Input: part model. Units: mm. Frame: model coordinates. Face numbers are marked on the shaded views. A direction names the side the tool comes from. Give positions to 0.01 mm unless a question says otherwise; leave off trailing zeros. Loops run counter-clockwise (first coordinate to the right, second up) from the corner with the lowest first, then second, coordinate; pieces in that order, holes last. Notation, with made-up numbers: M 26.25,-15 L 55.25,-15 A14 ccw 55.25,12 Z; hole C 28,-37.75 d1. An arc over 180 degrees is marked long. Return JSON: item names as keys, results as strings. Group by question number.
```python
from build123d import *

# Parameters (mm, degrees)
F0_R     = 20
F1_DEPTH = 60
F2_DEPTH = 40
F0_R_2   = 15
F3_DEPTH = 20


with BuildPart() as f1:
    # F0 (on Top) → F1 (new body)
    with BuildSketch(Plane.XY):
        with BuildLine():
            ThreePointArc((-46, -39.799497), (-20.335206, -26.832816), (-10, 0))
            ThreePointArc((-10, 0), (-20.335206, 26.832816), (-46, 39.799497))
            ThreePointArc((-46, 39.799497), (-90, 0), (-46, -39.799497))
        make_face()
        with Locations((-50, 0)):
            Circle(F0_R, mode=Mode.SUBTRACT)
    extrude(amount=F1_DEPTH)

    # F0 (on Top) → F2 (join)
    with BuildSketch(Plane.XY):
        with BuildLine():
            ThreePointArc((-46, 39.799497), (-20.335206, 26.832816), (-10, 0))
            ThreePointArc((-10, 0), (-20.335206, -26.832816), (-46, -39.799497))
            Line((-46, -39.799497), (53, -29.849623))
            ThreePointArc((53, -29.849623), (20, 0), (53, 29.849623))
            Line((53, 29.849623), (-46, 39.799497))
        make_face()
    extrude(amount=F2_DEPTH)

    # F0 (on Top) → F3 (join)
    with BuildSketch(Plane.XY):
        with BuildLine():
            ThreePointArc((80, 0), (72.248595, 20.124612), (53, 29.849623))
            ThreePointArc((53, 29.849623), (20, 0), (53, -29.849623))
            ThreePointArc((53, -29.849623), (72.248595, -20.124612), (80, 0))
        make_face()
        with Locations((50, 0)):
            Circle(F0_R_2, mode=Mode.SUBTRACT)
    extrude(amount=F3_DEPTH)


solid = f1.part
```
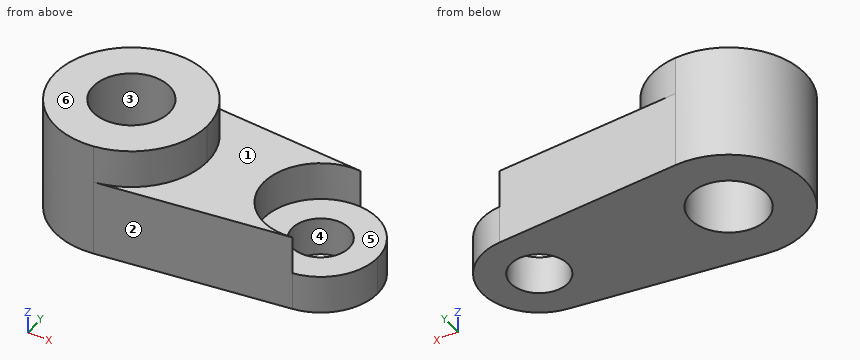
Item 1: Pull-direction query (X, two-part tool) for the marked faces 1, 2, 3 and 4; classes: pulls with the +X half, pulls with the -X half, needs draft (parallel to the pull), parting line crosses it, or undercut.
Item 2: Material intervals for line 1 (X direction, y = -13, z = 5); line 2 (Y direction, x = -50, z = 15); line 3 (Z direction, x = 4.5, y = 12), sorted ascending. Write a range as from..to.
Item 3: Section B-B, the plane x = -50. Return loops of the section in (y, z), then the cut area to 3 significant figures.
Item 4: Section A-A, the plane z = 17.5. Return loops of the section in (x, y), then the cut area to 3 significant figures.
Item 5: First-contact query: pin 1 Ø8 at (y, z) = (15.5, 27) entering from +X; pin 2 Ø10 at (x, y) = (23, 12.5) entering from +Z; pin 3 Ø1 at (x, z) = (-6, 32.5) entering from -Y. Flat tips, straight axial feed; report the tip coordinate or a pass-through.
Item 6: Reachability of the marked faces 5 and 6 from +Z, -Z, +X, -X, +Y, -Y: full face, straight path, thin tool, end or side. Return the list, or none.
Item 7: Section C-C, the plane y = 2. Return loops of the section in (x, z).
Item 8: Section D-D, the plane y = -12. Return loops of the section in (x, z), then the cut area to 3 significant figures.
Answer below:
{
 "1": {"face 1": "needs draft", "face 2": "pulls with the +X half", "face 3": "undercut", "face 4": "undercut"},
 "2": {"line 1": "-87.83..-65.2, -34.8..42.52, 57.48..77.04", "line 2": "-40..-20, 20..40", "line 3": "0..40"},
 "3": {"outline": "M -40,0 L -20,0 L -20,60 L -40,60 Z; M 20,0 L 40,0 L 40,60 L 20,60 Z", "area": "2,400 mm^2"},
 "4": {"outline": "M -46,-39.8 L 53,-29.85 A30 ccw 53,29.85 L -46,39.8 A40 ccw long Z; hole C -50,0 d40; hole C 50,0 d30", "area": "9,000 mm^2"},
 "5": {"pin 1": "x = 27.2", "pin 2": "z = 40", "pin 3": "y = -35.83"},
 "6": {"face 5": "+Z, +X", "face 6": "+Z, +X, -X, +Y, -Y"},
 "7": {"outline": "M -89.95,0 L -69.9,0 L -69.9,60 L -89.95,60 Z; M -30.1,0 L 35.13,0 L 35.13,20 L 20.07,20 L 20.07,40 L -10.05,40 L -10.05,60 L -30.1,60 Z; M 64.87,0 L 79.93,0 L 79.93,20 L 64.87,20 Z"},
 "8": {"outline": "M -88.16,0 L -66,0 L -66,60 L -88.16,60 Z; M -34,0 L 41,0 L 41,20 L 22.5,20 L 22.5,40 L -11.84,40 L -11.84,60 L -34,60 Z; M 59,0 L 77.5,0 L 77.5,20 L 59,20 Z", "area": "4,770 mm^2"}
}
